```python
from build123d import *

# Parameters (mm, degrees)
F0_W     = 25.98
F0_H     = 25.98
F1_DEPTH = 1
F2_R     = 5
F3_W     = 21.04
F3_H     = 21.04
F4_DEPTH = 1.5
F5_R     = 5


with BuildPart() as f1:
    # F0 (on Top) → F1 (new body)
    with BuildSketch(Plane.XY):
        Rectangle(F0_W, F0_H)
    extrude(amount=F1_DEPTH)

    # F2
    f2_edges = [f1.edges().sort_by_distance(p)[0] for p in [
        (-12.99, -12.99, 0.5),
        (12.99, -12.99, 0.5),
        (12.99, 12.99, 0.5),
        (-12.99, 12.99, 0.5),
    ]]
    fillet(f2_edges, radius=F2_R)

    # F3 (on face) → F4 (join)
    with BuildSketch(Plane(origin=(0, 0, 0), x_dir=(1, 0, 0), z_dir=(0, 0, -1))):
        Rectangle(F3_W, F3_H)
    extrude(amount=F4_DEPTH)

    # F5
    f5_edges = [f1.edges().sort_by_distance(p)[0] for p in [
        (10.52, -10.52, -0.75),
        (-10.52, -10.52, -0.75),
        (10.52, 10.52, -0.75),
        (-10.52, 10.52, -0.75),
    ]]
    fillet(f5_edges, radius=F5_R)


solid = f1.part
```
Geometry: final body of the model. Coordinates: model frame, mm. A direction names the side the tool comes from. Give positions to 0.01 mm unless a question says otherwise; leave off trailing zeros. Write each loop counter-clockwise with the first axis right and the second up, starting at its lowest first coordinate (ties: lowest second). Pieces come first, ordered by that corner, then holes.
1. Section query B-B, the plane z = 0.5. Return loops of the section in (x, y).
2. Pin query (flat end, axial travel): P1, Ø0.8, axis at x = 1, z = -0.5, coming from the +Y side; P2, Ø0.8, axis at x = -2.5, z = -1, coming from the -Y side; P3, Ø0.8, axis at y = -1.5, z = -1, coming from the +X side. Return the tip coordinate at first contact, or that it passes through.
3. Section query A-A, the plane x = 4.25. Return loops of the section in (y, z), then the cut area to 3 significant figures.
4. Reachability of faces 1 (the flat face through (-10.52, 0, -1)), 2 (the flat face through (0, 10.52, -1)), 3 (the cylindrical face through (9.09, 9.02, -0.76)), 4 (the cylindrical face through (9.02, -9.09, -0.76)) from +Z, -Z, +X, -X, +Y, -Y: full face, straight path, thin tool, end or side. Return the list, or none.
5. Line query: probe 1 along Y at (x, z) = (-5.25, -0.85); probe 2 along Z at (x, y) = (10.75, 4). Output: solid intervals per line, ascending.
Computed:
1. outline: (-12.99, -7.99) arc R5 ccw to (-7.99, -12.99) - (7.99, -12.99) arc R5 ccw to (12.99, -7.99) - (12.99, 7.99) arc R5 ccw to (7.99, 12.99) - (-7.99, 12.99) arc R5 ccw to (-12.99, 7.99) - close
2. P1: stops at y = 10.52
2. P2: stops at y = -10.52
2. P3: stops at x = 10.52
3. outline: (-12.99, 0) - (-10.52, 0) - (-10.52, -1.5) - (10.52, -1.5) - (10.52, 0) - (12.99, 0) - (12.99, 1) - (-12.99, 1) - close
3. area: 57.5 mm2
4. face 1: -Z, -X, +Y, -Y
4. face 2: -Z, +X, -X, +Y
4. face 3: -Z, +X, +Y
4. face 4: -Z, +X, -Y
5. probe 1: y = -10.52 to 10.52
5. probe 2: z = 0 to 1
